Check sheet for the modelled part. Datum: model origin and axes. Units: mm. Give positions to 0.01 mm unless a question says otherwise; leave off trailing zeros. Write each loop counter-clockwise with the first axis right and the second up, starting at its lowest first coordinate (ties: lowest second). Pieces come first, ordered by that corner, then holes. Notation, with made-up numbers: (26, -18.5) -> (54, -18.5) arc R25 ccw to (54, 13.5) -> close; hole circle Ø1 at (-28.75, 27). An arc over 180 degrees is marked (long way). Return JSON: item names as keys, results as strings.
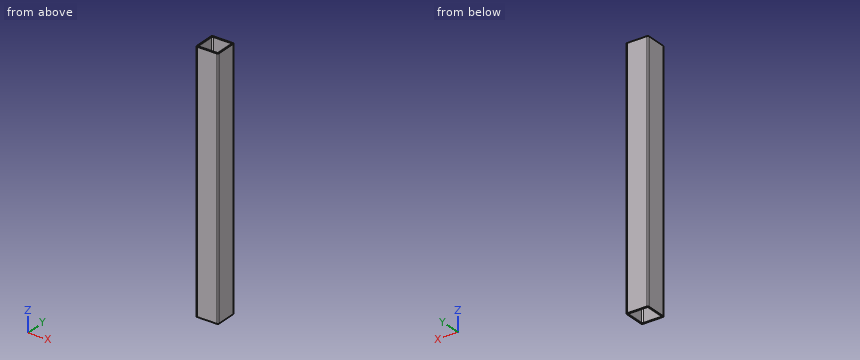
from build123d import *

# Parameters (mm, degrees)
DODANIE_WYCI_GNI_CIE1_DEPTH = 680


with BuildPart() as part:
    # Szkic1 → Dodanie-wyciągnięcie1 (new body)
    with BuildSketch(Plane.XY):
        with BuildLine():
            ThreePointArc((0, 57), (0.878679656, 59.121320344), (3, 60))
            Line((3, 60), (57, 60))
            ThreePointArc((57, 60), (59.121320344, 59.121320344), (60, 57))
            Line((60, 57), (60, 3))
            ThreePointArc((60, 3), (59.121320344, 0.878679656), (57, 0))
            Line((57, 0), (3, 0))
            ThreePointArc((3, 0), (0.878679656, 0.878679656), (0, 3))
            Line((0, 3), (0, 57))
        make_face()
        with BuildLine():
            Line((3, 6), (3, 54))
            ThreePointArc((3, 54), (3.878679656, 56.121320344), (6, 57))
            Line((6, 57), (54, 57))
            ThreePointArc((54, 57), (56.121320344, 56.121320344), (57, 54))
            Line((57, 54), (57, 6))
            ThreePointArc((57, 6), (56.121320344, 3.878679656), (54, 3))
            Line((54, 3), (6, 3))
            ThreePointArc((6, 3), (3.878679656, 3.878679656), (3, 6))
        make_face(mode=Mode.SUBTRACT)
    extrude(amount=DODANIE_WYCI_GNI_CIE1_DEPTH)


solid = part.part
(1) Cross-section at A-A on y = 23.5. Enter the section's corners in (x, z).
Reply:
{"outline": "(0, 0) -> (3, 0) -> (3, 680) -> (0, 680) -> close; (57, 0) -> (60, 0) -> (60, 680) -> (57, 680) -> close"}
(2) Cross-section at C-C on z = 221. Enter the section's corners in (x, y).
Reply:
{"outline": "(0, 3) arc R3 ccw to (3, 0) -> (57, 0) arc R3 ccw to (60, 3) -> (60, 57) arc R3 ccw to (57, 60) -> (3, 60) arc R3 ccw to (0, 57) -> close; hole (3, 6) arc R3 ccw to (6, 3) -> (54, 3) arc R3 ccw to (57, 6) -> (57, 54) arc R3 ccw to (54, 57) -> (6, 57) arc R3 ccw to (3, 54) -> close"}
(3) Thickness scan on L1, parallel to Y at x = 43, z = 245.5; L2, parallel to X at y = 5, z = 337. Record the ranges inside material, lowest first.
Reply:
{"L1": "0 to 3, 57 to 60", "L2": "0 to 3.17, 56.83 to 60"}
